Part print with two shaded views. Sizes in mm from the minimum x, y, z corner. A direction names the side the tool comes from. Coordinates: 2 decimals unless noted, no trailing zeros. Loops run counter-clockwise (first coordinate to the right, second up) from the corner with the lowest first, then second, coordinate; pieces in that order, holes last. Notation, with made-up numbers: (-31, 27.5) -> (8, 27.5) arc R7 ccw to (8, 40.5) -> close; hole circle Ø5 at (73, 34). An arc over 180 degrees is marked (long way). Return JSON: item names as keys, results as strings. Group by question number.
(1) Probe L1, parallel to X at y = 9, z = 20.5; L2, parallel to Y at x = 29, z = 19; L3, parallel to Y at x = 21, z = 16. List the from-to ranges inside material, lowest first.
(2) Tool access for the marked faces 1 and 2: list every direction of +Z, -Z, +X, -X, +Y, -Y with a clear straight run to the whole face (end or side of a thin tool).
(3) Mould opens along X. For the marked faces 3, 4, 5 and 6 say: pulls with the +X half, pulls with the -X half, needs draft (parallel to the pull), parting line crosses it, or undercut.
(4) Saw through at B-B on z = 19. Write the cut outline in (x, y), then the cut area to 3 significant figures.
(5) Saw through at C-C on z = 27. Write the cut outline in (x, y).
(6) Saw through at A-A on y = 16.7. Write the cut outline in (x, z).
(7) Saw through at D-D on y = 36.5. Write the cut outline in (x, z), then the cut area to 3 significant figures.
(8) Flat gauge pins, fed straight in: pin 1 Ø5 at (x, y) = (18, 8) entering from -Z; pin 2 Ø6 at (x, z) = (15, 15.5) entering from +Y. Where does each tip first touch, or does it go through?
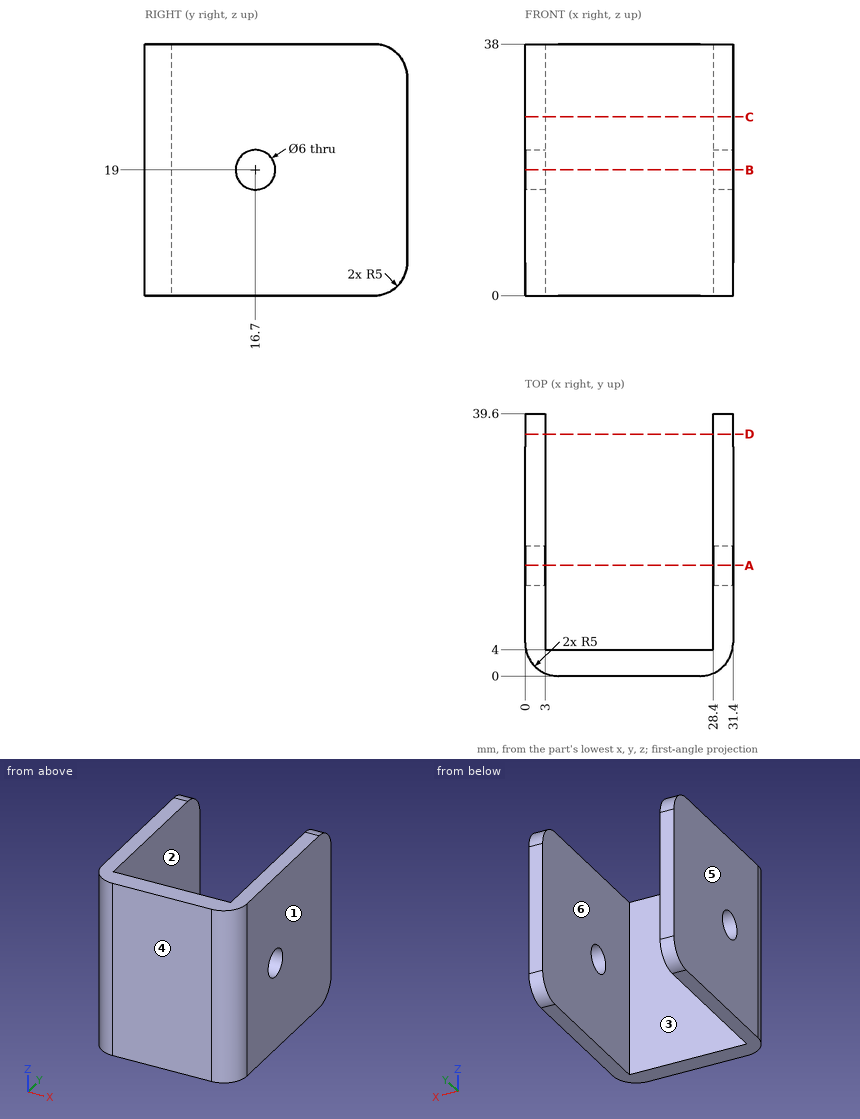
Geometry results:
{
 "1": {"L1": "0 to 3, 28.4 to 31.4", "L2": "0.73 to 13.7, 19.7 to 39.6", "L3": "0 to 4"},
 "2": {"face 1": "+Z, -Z, +X, +Y, -Y", "face 2": "+Z, -Z, +Y"},
 "3": {"face 3": "undercut", "face 4": "needs draft", "face 5": "pulls with the -X half", "face 6": "undercut"},
 "4": {"outline": "(0, 5) arc R5 ccw to (5, 0) -> (26.4, 0) arc R5 ccw to (31.4, 5) -> (31.4, 13.7) -> (28.4, 13.7) -> (28.4, 4) -> (3, 4) -> (3, 13.7) -> (0, 13.7) -> close; (0, 19.7) -> (3, 19.7) -> (3, 39.6) -> (0, 39.6) -> close; (28.4, 19.7) -> (31.4, 19.7) -> (31.4, 39.6) -> (28.4, 39.6) -> close", "area": "292 mm²"},
 "5": {"outline": "(0, 5) arc R5 ccw to (5, 0) -> (26.4, 0) arc R5 ccw to (31.4, 5) -> (31.4, 39.6) -> (28.4, 39.6) -> (28.4, 4) -> (3, 4) -> (3, 39.6) -> (0, 39.6) -> close"},
 "6": {"outline": "(0, 0) -> (3, 0) -> (3, 16) -> (0, 16) -> close; (0, 22) -> (3, 22) -> (3, 38) -> (0, 38) -> close; (28.4, 0) -> (31.4, 0) -> (31.4, 16) -> (28.4, 16) -> close; (28.4, 22) -> (31.4, 22) -> (31.4, 38) -> (28.4, 38) -> close"},
 "7": {"outline": "(0, 0.38) -> (3, 0.38) -> (3, 37.62) -> (0, 37.62) -> close; (28.4, 0.38) -> (31.4, 0.38) -> (31.4, 37.62) -> (28.4, 37.62) -> close", "area": "223 mm²"},
 "8": {"pin 1": "through", "pin 2": "y = 4"}
}
